Input: part model. Units: mm. Frame: model coordinates. Face numbers are marked on the shaded views. A direction names the side the tool comes from. Coordinates: 2 decimals unless noted, no trailing zeros. Loops run counter-clockwise (first coordinate to the right, second up) from the corner with the lowest first, then second, coordinate; pieces in that order, holes last. Notation, with made-up numbers: M 38,-38.5 L 50,-38.5 A28 cw 50,-11.5 Z; hole C 73,-26.5 d4. An arc over 180 degrees is marked long. Use a Markdown table: item, result. Add a question column.
1. Section D-D on x = -5. Output: boundary loops of the cut face in (y, z), then the cut area to 3 significant figures.
2. Section A-A on x = 1.5. Output: boundary loops of the cut face in (y, z).
3. Pin query (flat end, axial travel): pin 1 (1.4 mm diameter, centred on y = 2, z = 15.5, fed in from -X); pin 2 (2.5 mm diameter, centred on y = 1.5, z = -14, fed in from -X); pin 3 (0.5 mm diameter, centred on y = 5.5, z = 0.5, fed in from -X); pin 4 (3 mm diameter, centred on x = 17.5, y = 1.5, fed in from -Z). Return the tip coordinate at first contact, or that it passes through.
4. Section C-C on z = -10. Output: boundary loops of the cut face in (x, y), then the cut area to 3 significant figures.
5. Section B-B on y = 2.5. State how many separate pieces and enclosed holes the cut face has, then the cut area to 3 significant figures.
6. Draft query along X for the marked faces 1, 2 and 3. Return one class per face: +X half, -X half, draft (parallel to the pull), parting line (faces both ways), or undercut.
7. Set-up query: the marked faces 4, 5 and 6. Return all of +Z, -Z, +X, -X, +Y, -Y with unobstructed straight access to the full face (end or side cutting, diameter ignored); none if empty.
8. Line query: L1, parallel to Z at x = 0.5, y = 3.65; L2, parallel to X at y = 3.9, z = 13.5; L3, parallel to Z at x = -15, y = 3.75. Output: solid intervals per line, ascending. Write a range as [from, to].
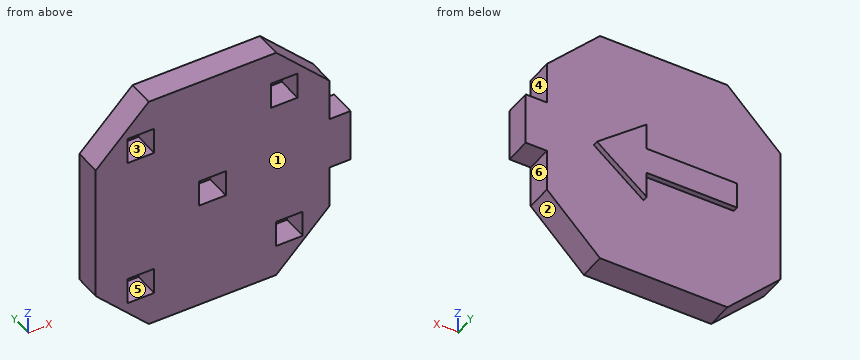
```python
from build123d import *

# Parameters (mm, degrees)
BOSS_EXTRU_1_DEPTH      = 5
BOSS_EXTRU_2_DEPTH      = 1
ESQUISSE3_W             = 5
ESQUISSE3_H             = 5
ENL_V_MAT_EXTRU_1_DEPTH = 4.8


with BuildPart() as part:
    # Esquisse1 → Boss.-Extru.1 (new body)
    with BuildSketch(Plane(origin=(0, 0, 0), x_dir=(1, 0, 0), z_dir=(0, 1, 0))):
        Polygon((22, 13), (12.003020456, 23), (-12.003020456, 23), (-22, 13), (-22, -13), (-12.003020456, -23), (12.003020456, -23), (22, -13), (22, -5), (26, -5), (26, 5), (22, 5), align=None)
    extrude(amount=BOSS_EXTRU_1_DEPTH)

    # Esquisse2 → Boss.-Extru.2 (add)
    with BuildSketch(Plane(origin=(0, 5, 0), x_dir=(1, 0, 0), z_dir=(0, 1, 0))):
        Polygon((3.82, 2.552581319), (3.82, 7.552581319), (13.187496998, 0.052581319), (3.82, -7.447418681), (3.82, -2.447418681), (-13.18, -2.447418681), (-13.18, 2.552581319), align=None)
    extrude(amount=BOSS_EXTRU_2_DEPTH)

    # Esquisse3 → Enlèv. mat.-Extru.1 (cut)
    with BuildSketch(Plane.XZ):
        with Locations((-13.5, 14.5)):
            Rectangle(ESQUISSE3_W, ESQUISSE3_H)
        with Locations((-13.5, -14.5)):
            Rectangle(ESQUISSE3_W, ESQUISSE3_H)
        with Locations((14.5, -14.5)):
            Rectangle(ESQUISSE3_W, ESQUISSE3_H)
        with Locations((13.5, 14.5)):
            Rectangle(ESQUISSE3_W, ESQUISSE3_H)
        Rectangle(ESQUISSE3_W, ESQUISSE3_H)
    extrude(amount=-ENL_V_MAT_EXTRU_1_DEPTH, mode=Mode.SUBTRACT)


solid = part.part
```
Answers below:
| question | item | result |
|---|---|---|
| 1 | outline | M 0,-23 L 5,-23 L 5,-2.55 L 6,-2.55 L 6,2.45 L 5,2.45 L 5,23 L 0,23 Z |
| 1 | area | 235 mm² |
| 2 | outline | M 0,-23 L 5,-23 L 5,-2.55 L 6,-2.55 L 6,2.45 L 5,2.45 L 5,23 L 0,23 L 0,2.5 L 4.8,2.5 L 4.8,-2.5 L 0,-2.5 Z |
| 3 | pin 1 | stops at x = -20.2 |
| 3 | pin 2 | stops at x = -22 |
| 3 | pin 3 | stops at x = -13.18 |
| 3 | pin 4 | stops at z = -19 |
| 4 | outline | M -22,0 L 22,0 L 22,5 L -22,5 Z |
| 4 | area | 220 mm² |
| 5 | separate pieces | 1 |
| 5 | enclosed holes | 5 |
| 5 | area | 1,740 mm² |
| 6 | face 1 | draft |
| 6 | face 2 | +X half |
| 6 | face 3 | undercut |
| 7 | face 4 | +Z, +X, +Y, -Y |
| 7 | face 5 | -Y |
| 7 | face 6 | -Z, +X, +Y, -Y |
| 8 | L1 | z = [-23, -2.5], [2.5, 23] |
| 8 | L2 | x = [-21.5, -16], [-11, 11], [16, 21.5] |
| 8 | L3 | z = [-20, -17], [-12, 12], [17, 20] |
